Part print with two shaded views. Sizes in mm from the minimum x, y, z corner. A direction names the side the tool comes from. Give positions to 0.01 mm unless a question says otherwise; leave off trailing zeros. Order: outer loops, then holes, each group sorted by start corner. A loop starts at its lowest first (then second) coordinate and runs counter-clockwise, first axis right, second up. Notation, with made-up numbers: M 40.5,33.25 L 70.5,33.25 A33 ccw 70.5,61.25 Z; hole C -18,19.25 d10. An arc over 180 degrees is marked long. Return JSON: item names as keys, results as strings.
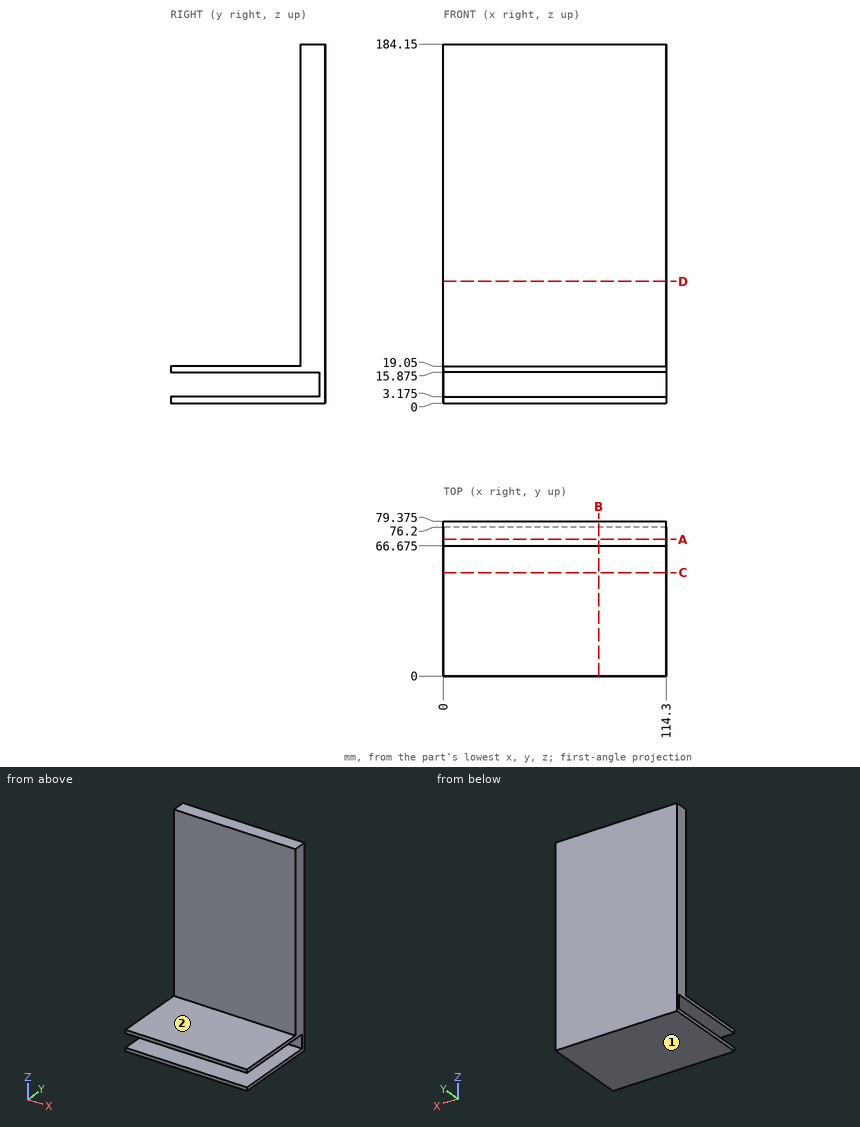
Q1. Band-saw the part on D-D (z = 62.5). Give the cut face in (x, y) (3 decimals), then the cut area to 3 significant figures.
Established:
{"outline": "M 0,66.675 L 114.3,66.675 L 114.3,79.375 L 0,79.375 Z", "area": "1,450 mm²"}
Q2. Band-saw the part on B-B (x = 79.5). Give the cut face in (y, z) (3 decimals).
Established:
{"outline": "M 0,0 L 79.375,0 L 79.375,184.15 L 66.675,184.15 L 66.675,19.05 L 0,19.05 L 0,15.875 L 76.2,15.875 L 76.2,3.175 L 0,3.175 Z"}
Q3. Pin check, flat tips, straight feed: pin 1 (3 mm diameter, centred on x = 88, z = 50, fed in from -Y) (3 decimals); pin 2 (6.5 mm diameter, centred on x = 35, z = 11.5, fed in from -Y); pin 3 (1 mm diameter, centred on y = 65, z = 84.5, fed in from -X); pin 4 (1 mm diameter, centred on x = 30, y = 28, fed in from -Z). Stop position of each tip, or through.
Established:
{"pin 1": "stops at y = 66.675", "pin 2": "stops at y = 76.2", "pin 3": "passes through", "pin 4": "stops at z = 0"}
Q4. Band-saw the part on C-C (y = 53). Give the cut face in (x, z) (3 decimals), then the cut area to 3 significant figures.
Established:
{"outline": "M 0,0 L 114.3,0 L 114.3,3.175 L 0,3.175 Z; M 0,15.875 L 114.3,15.875 L 114.3,19.05 L 0,19.05 Z", "area": "726 mm²"}
Q5. 3-axis set-ups, long thin cutter, end or side, ignore diameter. For the marked faces 1 and 2: which of +Z, -Z, +X, -X, +Y, -Y reach the whole face in a straight line?
Established:
{"face 1": "-Z, +X, -X, +Y, -Y", "face 2": "+Z, +X, -X, -Y"}
Q6. Band-saw the part on A-A (y = 70). Give the cut face in (x, z) (3 decimals).
Established:
{"outline": "M 0,0 L 114.3,0 L 114.3,3.175 L 0,3.175 Z; M 0,15.875 L 114.3,15.875 L 114.3,184.15 L 0,184.15 Z"}
Q7. Probe line 1 along Z through (x, y) = (75, 24) (3 decimals); line 2 along Y through (x, z) = (101.5, 147.5) (3 decimals). List the from-to ranges inside material, lowest first.
Established:
{"line 1": "z = 0 to 3.175, 15.875 to 19.05", "line 2": "y = 66.675 to 79.375"}
